```python
from build123d import *

# Parameters (mm, degrees)
SKETCH_W      = 226
SKETCH_H      = 56
PAD_DEPTH     = 3
SKETCH001_R   = 5.5
SKETCH001_W   = 20
SKETCH001_H   = 3
SKETCH001_W_2 = 3
SKETCH001_H_2 = 8
POCKET_DEPTH  = 5


with BuildPart() as part:
    # Sketch → Pad (new body)
    with BuildSketch(Plane.XY):
        with Locations((113, 28)):
            Rectangle(SKETCH_W, SKETCH_H)
    extrude(amount=PAD_DEPTH)

    # Sketch001 (on Face6 of Pad) → Pocket (cut)
    with BuildSketch(Plane.XY.offset(3)):
        with Locations((31, 26.5)):
            Circle(SKETCH001_R)
        with Locations((33, 4.5)):
            Rectangle(SKETCH001_W, SKETCH001_H)
        with Locations((73, 4.5)):
            Rectangle(SKETCH001_W, SKETCH001_H)
        with Locations((113, 4.5)):
            Rectangle(SKETCH001_W, SKETCH001_H)
        with Locations((153, 4.5)):
            Rectangle(SKETCH001_W, SKETCH001_H)
        with Locations((193, 4.5)):
            Rectangle(SKETCH001_W, SKETCH001_H)
        with Locations((33, 17.5)):
            Rectangle(SKETCH001_W, SKETCH001_H)
        with Locations((73, 17.5)):
            Rectangle(SKETCH001_W, SKETCH001_H)
        with Locations((113, 17.5)):
            Rectangle(SKETCH001_W, SKETCH001_H)
        with Locations((153, 17.5)):
            Rectangle(SKETCH001_W, SKETCH001_H)
        with Locations((193, 17.5)):
            Rectangle(SKETCH001_W, SKETCH001_H)
        with Locations((33, 51.5)):
            Rectangle(SKETCH001_W, SKETCH001_H)
        with Locations((73, 51.5)):
            Rectangle(SKETCH001_W, SKETCH001_H)
        with Locations((113, 51.5)):
            Rectangle(SKETCH001_W, SKETCH001_H)
        with Locations((153, 51.5)):
            Rectangle(SKETCH001_W, SKETCH001_H)
        with Locations((193, 51.5)):
            Rectangle(SKETCH001_W, SKETCH001_H)
        with Locations((4.5, 12)):
            Rectangle(SKETCH001_W_2, SKETCH001_H_2)
        with Locations((4.5, 28)):
            Rectangle(SKETCH001_W_2, SKETCH001_H_2)
        with Locations((4.5, 44)):
            Rectangle(SKETCH001_W_2, SKETCH001_H_2)
        with Locations((221.5, 12)):
            Rectangle(SKETCH001_W_2, SKETCH001_H_2)
        with Locations((221.5, 28)):
            Rectangle(SKETCH001_W_2, SKETCH001_H_2)
        with Locations((221.5, 44)):
            Rectangle(SKETCH001_W_2, SKETCH001_H_2)
    extrude(amount=-POCKET_DEPTH, mode=Mode.SUBTRACT)


solid = part.part
```
The model under review builds one solid part; all positions refer to its coordinate system, in mm. Round coordinates to 2 decimals unless told otherwise and drop trailing zeros. Order: outer loops, then holes, each group sorted by start corner. A loop starts at its lowest first (then second) coordinate and runs counter-clockwise, first axis right, second up. Notation, with made-up numbers: (50.5, 32.5) -> (60.5, 32.5) arc R11 ccw to (60.5, 46.5) -> close; hole circle Ø7 at (-35.5, -34). An arc over 180 degrees is marked (long way). Use a Markdown table: item, result.
Q1. We need section A-A on y = 26.5. Write out the cut boundary in (x, z).
Values:
| item | result |
|---|---|
| outline | (0, 0) -> (3, 0) -> (3, 3) -> (0, 3) -> close; (6, 0) -> (25.5, 0) -> (25.5, 3) -> (6, 3) -> close; (36.5, 0) -> (220, 0) -> (220, 3) -> (36.5, 3) -> close; (223, 0) -> (226, 0) -> (226, 3) -> (223, 3) -> close |
Q2. Mouldability with a two-part tool opening along X and no side actions: class faces 1 (the cylindrical face through (26.95, 30.22, 1.52)), 2 (the flat face through (111, 28, 3)) as +X half, -X half, draft (parallel to the pull), parting line (faces both ways), or undercut.
Values:
| item | result |
|---|---|
| face 1 | undercut |
| face 2 | draft |
Q3. For line 1 (Y direction, x = 31, z = 1.25); line 2 (Y direction, x = 66, z = 1); line 3 (X direction, y = 45.5, z = 2.15), list the stretches that pass through material, from the lowest coordinate up.
Values:
| item | result |
|---|---|
| line 1 | y = 0 to 3, 6 to 16, 19 to 21, 32 to 50, 53 to 56 |
| line 2 | y = 0 to 3, 6 to 16, 19 to 50, 53 to 56 |
| line 3 | x = 0 to 3, 6 to 220, 223 to 226 |
Q4. We need section C-C on z = 1.75. State how many separate pieces and enclosed holes the cut face has, then the cut area to 3 significant figures.
Values:
| item | result |
|---|---|
| separate pieces | 1 |
| enclosed holes | 22 |
| area | 11,500 mm^2 |
Q5. We need section B-B on x = 31. Write out the cut boundary in (y, z).
Values:
| item | result |
|---|---|
| outline | (0, 0) -> (3, 0) -> (3, 3) -> (0, 3) -> close; (6, 0) -> (16, 0) -> (16, 3) -> (6, 3) -> close; (19, 0) -> (21, 0) -> (21, 3) -> (19, 3) -> close; (32, 0) -> (50, 0) -> (50, 3) -> (32, 3) -> close; (53, 0) -> (56, 0) -> (56, 3) -> (53, 3) -> close |
